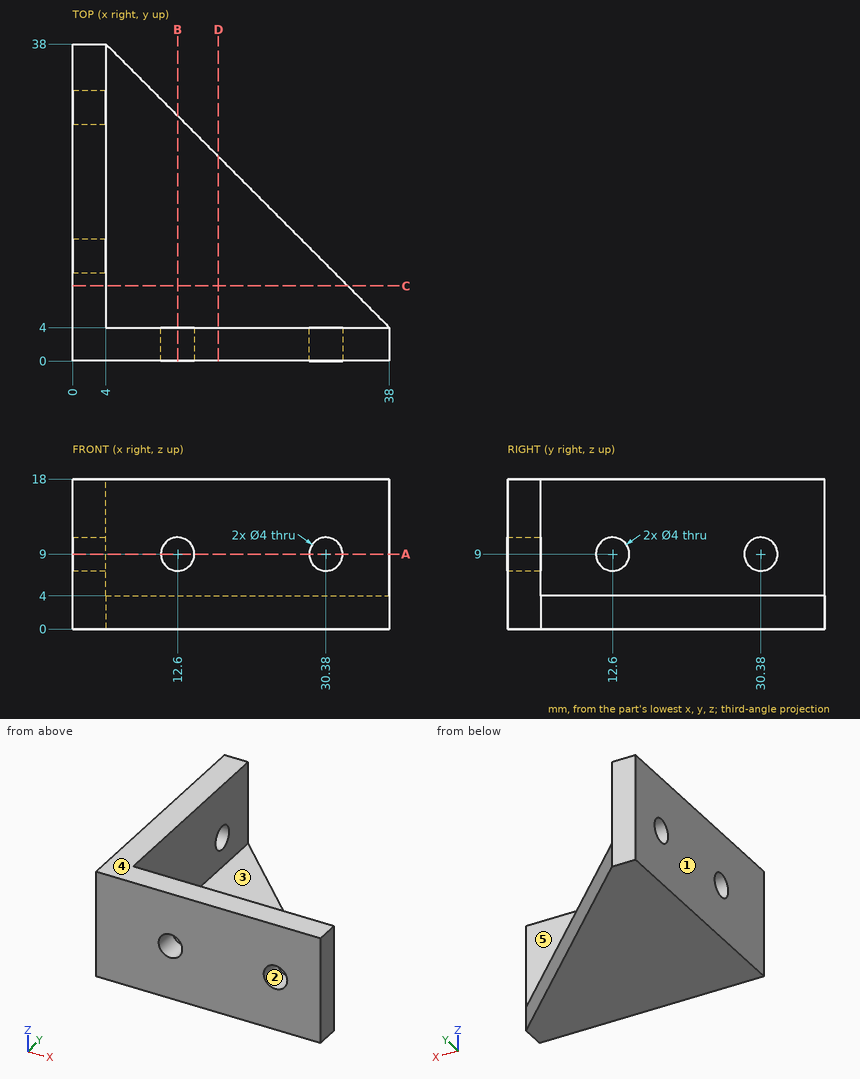
Could you check a few things on this drawing? It's one solid part, dimensions in mm from its lowest x, y, z. A direction names the side the tool comes from. Give positions to 0.01 mm unless a question says otherwise; leave off trailing zeros. Write each loop counter-clockwise with the first axis right and the second up, starting at its lowest first coordinate (ties: lowest second). Pieces come first, ordered by that corner, then holes.
(1) Will these pins go through, and if not, where does the flat tip stop? pin 1 (5 mm diameter, centred on y = 13.5, z = 4.5, fed in from +X); pin 2 (3 mm diameter, centred on x = 27, z = 10, fed in from +Y); pin 3 (8 mm diameter, centred on y = 18.5, z = 15, fed in from +X).
Output values:
pin 1: stops at x = 30.95
pin 2: stops at y = 4
pin 3: stops at x = 4
(2) Imagine slicing it at D-D, the plane x = 17.5. Write out the boundary of the cut face in (y, z).
Output values:
outline: (0, 0) - (24.5, 0) - (24.5, 4) - (4, 4) - (4, 18) - (0, 18) - close
(3) If I drill on L1, parallel to Z at x = 0.8, y = 12.6; L2, parallel to Y at x = 9.5, z = 7.5; L3, parallel to Z at x = 2, y = 12, over which ranges is the centre line in solid material (lowest first)?
Output values:
L1: z = 0 to 7, 11 to 18
L2: y = 0 to 4
L3: z = 0 to 7.09, 10.91 to 18
(4) Thinking about a two-plate mould opening in X: for the marked faces 1, 2 and 3, which applies, pulls with the +X half, pulls with the -X half, needs draft (parallel to the pull), parting line crosses it, or undercut?
Output values:
face 1: pulls with the -X half
face 2: undercut
face 3: needs draft
(5) Imagine slicing it at C-C, the plane y = 9. Write out the boundary of the cut face in (x, z).
Output values:
outline: (0, 0) - (33, 0) - (33, 4) - (4, 4) - (4, 18) - (0, 18) - close
(6) Imagine slicing it at B-B, the plane x = 12.6. Write out the boundary of the cut face in (y, z), and give its area (3 significant figures).
Output values:
outline: (0, 0) - (29.4, 0) - (29.4, 4) - (4, 4) - (4, 7) - (0, 7) - close; (0, 11) - (4, 11) - (4, 18) - (0, 18) - close
area: 158 mm2
(7) Imagine slicing it at A-A, the plane z = 9. Write out the boundary of the cut face in (x, y).
Output values:
outline: (0, 0) - (10.6, 0) - (10.6, 4) - (4, 4) - (4, 10.6) - (0, 10.6) - close; (0, 14.6) - (4, 14.6) - (4, 28.38) - (0, 28.38) - close; (0, 32.38) - (4, 32.38) - (4, 38) - (0, 38) - close; (14.6, 0) - (28.38, 0) - (28.38, 4) - (14.6, 4) - close; (32.38, 0) - (38, 0) - (38, 4) - (32.38, 4) - close
(8) On a 3-axis mill with a long thin cutter (end or side, diameter ignored), from which of +Z, -Z, +X, -X, +Y, -Y can I reach the whole of each face in a straight line? I mean the marked faces 4 and 5. Say none if no direction works.
Output values:
face 4: +Z, +X, -X, +Y, -Y
face 5: +Z, +X, +Y
